The listing builds one solid part. Answer for the finished solid, in the listing's coordinates (mm). Face numbers are marked on the shaded views. A direction names the side the tool comes from. Coordinates: 2 decimals unless noted, no trailing zeros. Order: outer loops, then holes, each group sorted by start corner. A loop starts at its lowest first (then second) coordinate and runs counter-clockwise, first axis right, second up. Notation, with made-up numbers: (-15.75, -20.75) - (25.25, -20.75) arc R23 cw to (25.25, -11.75) - close; hole circle Ø5 at (-17.5, 78.5). An arc over 180 degrees is marked (long way). Use one line per item in the form item = value. Start each with the question number.
Item 1: Section A-A, the plane z = 15 is taken. Write down the section's boundary in (x, y).
Item 2: Section B-B, the plane y = -79 is taken. Write down the section's boundary in (x, z).
Item 3: Section D-D, the plane y = -107.5 is taken. Write down the section's boundary in (x, z), and give its area (3 significant figures).
Item 4: The mould has two halves that part along Y. Classify the marked faces 4, 5 and 6: released by +Y, released by -Y, zero draft, split by the parting line, or undercut.
Item 5: Each of these flat-tipped pins is pushed along its axis until it touches: pin 1 Ø4.5 at (x, z) = (-2, -23) entering from -Y; pin 2 Ø2 at (x, z) = (3.5, -30) entering from -Y; pin 3 Ø1.2 at (x, z) = (3.5, -27.5) entering from +Y. Where does it stop, or does it pass through?
Item 6: Section C-C, the plane y = -181.5 is taken. Write down the section's boundary in (x, z), and give its area (3 significant figures).
Item 7: Consider line 1 along Y through (x, z) = (-2, 20.5); line 2 along Y through (x, z) = (-3.5, 15); line 3 along Z through (x, y) = (0, -16). Determine where each line is inside the solid, lowest interval first. Write a range as [from, to].
Item 8: A tool of negligible diameter and unlimited length cuts with its end or side. For the marked faces 1, 2 and 3, from which of +Z, -Z, +X, -X, +Y, -Y can it reach the whole face along a straight path? Write none if from no direction.
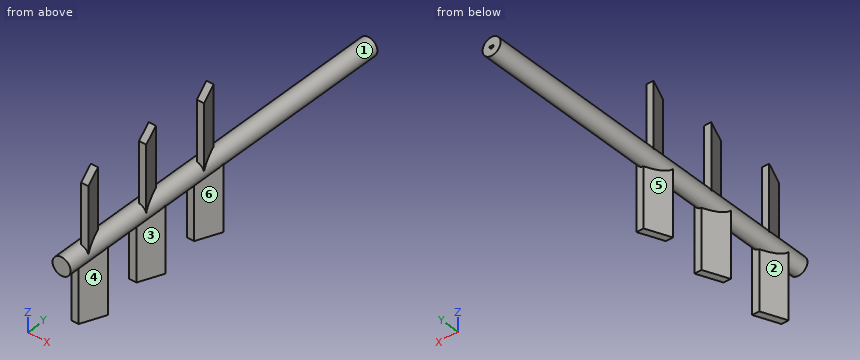
from build123d import *

# Parameters (mm, degrees)
F0_R     = 5
F1_DEPTH = 203.2
F3_DEPTH = 38.1
F5_DEPTH = 38.1
F7_DEPTH = 10


with BuildPart() as f1:
    # F0 (on Front) → F1 (new body)
    with BuildSketch(Plane.XZ):
        Circle(F0_R)
    extrude(amount=F1_DEPTH)

    # F2 (on Top) → F3 (join)
    with BuildSketch(Plane.XY):
        Polygon((0.735118, -114.487068), (4.735118, -114.487068), (-0.735118, -101.6), (-4.735118, -101.6), align=None)
        Polygon((4.735118, -152.774136), (-0.735118, -139.887068), (-4.735118, -139.887068), (0.735118, -152.774136), align=None)
        Polygon((4.735118, -191.061204), (-0.735118, -178.174136), (-4.735118, -178.174136), (0.735118, -191.061204), align=None)
    extrude(amount=F3_DEPTH)

    # F4 (on Top) → F5 (join)
    with BuildSketch(Plane.XY):
        Polygon((-4.735118, -114.487068), (-0.735118, -114.487068), (4.735118, -101.6), (0.735118, -101.6), align=None)
        Polygon((-4.735118, -152.774136), (-0.735118, -152.774136), (4.735118, -139.887068), (0.735118, -139.887068), align=None)
        Polygon((-4.735118, -191.061204), (-0.735118, -191.061204), (4.735118, -178.174136), (0.735118, -178.174136), align=None)
    extrude(amount=-F5_DEPTH)

    # F6 (on Front) → F7 (cut)
    with BuildSketch(Plane.XZ):
        with BuildLine():
            Line((1, 0.416667), (-1, 0.416667))
            ThreePointArc((-1, 0.416667), (0, -1.083333), (1, 0.416667))
        make_face()
    extrude(amount=F7_DEPTH, mode=Mode.SUBTRACT)


solid = f1.part
Response:
q1.outline = (-4.74, -178.17) - (0.74, -191.06) - (4.74, -191.06) - (-0.74, -178.17) - close; (-4.74, -139.89) - (0.74, -152.77) - (4.74, -152.77) - (-0.74, -139.89) - close; (-4.74, -101.6) - (0.74, -114.49) - (4.74, -114.49) - (-0.74, -101.6) - close
q2.outline = circle Ø10 at (0, 0)
q3.outline = (-2.23, 4.47) arc R5 ccw to (-1.77, -4.68) - (-1.77, -38.1) - (2.23, -38.1) - (2.23, -4.47) arc R5 ccw to (1.77, 4.68) - (1.77, 38.1) - (-2.23, 38.1) - close
q3.area = 344 mm2
q4.face_4 = released by -Y
q4.face_5 = released by +Y
q4.face_6 = undercut
q5.pin_1 = -191.06
q5.pin_2 = -183.44
q5.pin_3 = -101.6
q6.outline = (-3.32, 3.74) arc R5 ccw to (-0.68, -4.95) - (-0.68, -38.1) - (3.32, -38.1) - (3.32, -3.74) arc R5 ccw to (0.68, 4.95) - (0.68, 38.1) - (-3.32, 38.1) - close
q6.area = 346 mm2
q7.line_1 = [-184.62, -178.17], [-146.33, -139.89], [-108.04, -101.6]
q7.line_2 = [-181.08, -178.17], [-142.8, -139.89], [-104.51, -101.6]
q7.line_3 = [-5, 5]
q8.face_1 = none
q8.face_2 = -Z, -X
q8.face_3 = -Z, +X
